Autodesk Inventor part; units mm, degrees
ref_plane "YZ Plane" through (0, 0, 0) normal (1, 0, 0) x (0, 1, 0)
ref_plane "XZ Plane" through (0, 0, 0) normal (0, 1, 0) x (-1, 0, 0)
ref_plane "XY Plane" through (0, 0, 0) normal (0, 0, 1) x (1, 0, 0)
sketch "Sketch1" plane through (0, 0, 0) normal (0, 1, 0) x (-1, 0, 0)
  line L0 (0, 0) -> (8, 0)
  line L1 (8, 0) -> (8, -50)
  line L2 (8, -50) -> (0, -50)
  line L3 (0, -50) -> (0, 0)
  line L4 (8, 0) -> (4, 0)
  line L5 (4, 0) -> (4, -4)
  circle A0 centre (4, -4) radius 2
  line L6 (8, -50) -> (4, -50)
  line L7 (4, -50) -> (4, -46)
  circle A1 centre (4, -46) radius 2
  dimension "d0" = 8
  dimension "d1" = 50
  dimension "d2" = 4
  dimension "d3" = 4
  dimension "d4" = 4
  dimension "d5" = 4
  dimension "d6" = 4
  dimension "d7" = 4
extrude "Extrusion1" add sketch "Sketch1" along normal blind 5
fillet "Fillet1" radius 4 4 edges at (0, 2.5, 0) (-8, 2.5, 0) (-8, 2.5, -50) (0, 2.5, -50)
properties part number "Bar2"
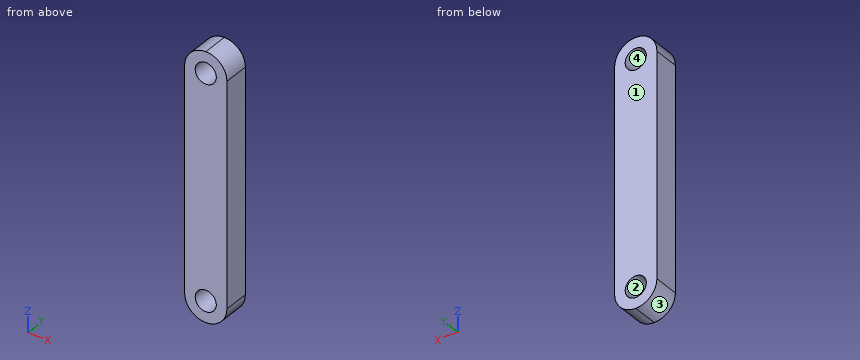
Here's how the part is built. I have some questions about the finished solid (model axes, mm). Face numbers are marked on the shaded views. Give positions to 0.01 mm unless a question says otherwise; leave off trailing zeros. Order: outer loops, then holes, each group sorted by start corner. A loop starts at its lowest first (then second) coordinate and runs counter-clockwise, first axis right, second up. Notation, with made-up numbers: (26.25, -7) - (73.25, -7) arc R21 ccw to (73.25, 4) - close; hole circle Ø11 at (71, -4). An arc over 180 degrees is marked (long way). Answer as a JSON object with one key per item and string values. Group by question number.
Item 1: Please list where these lines run through material, in increasing order: probe 1 along Z at (x, y) = (-4, 3.25); probe 2 along Z at (x, y) = (-5, 3.5); probe 3 along X at (y, z) = (3.05, -4).
Item 2: If we section it at B-B on y = 2.85: Give the number of separate pieces and of enclosed holes in the cut face, and give its area (3 significant figures).
Item 3: If we mould it in two halves opening along Z, with no side actions, what happens to the marked faces 1, 2, 3 and 4? For each: pulls with the +Z half, pulls with the -Z half, needs draft (parallel to the pull), parting line crosses it, or undercut.
Item 4: If we section it at C-C on x = -3: Please give me the cut outline in (y, z), and give its area (3 significant figures).
Item 5: For P1, Ø1, axis at x = -7, z = -29.5, coming from the -Y side; P2, Ø2, axis at x = -2, y = 3.5, coming from the +Z side, each with a flat end and sliding along its axis, tell me the tip position at first contact or that it passes through.
Item 6: If we section it at A-A on x = -5.25: Please give me the cut outline in (y, z).
Result set:
{
 "1": {"probe 1": "-50 to -48, -44 to -6, -2 to 0", "probe 2": "-49.87 to -47.73, -44.27 to -5.73, -2.27 to -0.13", "probe 3": "-8 to -6, -2 to 0"},
 "2": {"separate pieces": "1", "enclosed holes": "2", "area": "361 mm²"},
 "3": {"face 1": "needs draft", "face 2": "undercut", "face 3": "pulls with the -Z half", "face 4": "undercut"},
 "4": {"outline": "(0, -49.87) - (5, -49.87) - (5, -47.73) - (0, -47.73) - close; (0, -44.27) - (5, -44.27) - (5, -5.73) - (0, -5.73) - close; (0, -2.27) - (5, -2.27) - (5, -0.13) - (0, -0.13) - close", "area": "214 mm²"},
 "5": {"P1": "y = 0", "P2": "z = -0.13"},
 "6": {"outline": "(0, -49.8) - (5, -49.8) - (5, -47.56) - (0, -47.56) - close; (0, -44.44) - (5, -44.44) - (5, -5.56) - (0, -5.56) - close; (0, -2.44) - (5, -2.44) - (5, -0.2) - (0, -0.2) - close"}
}
